```python
from build123d import *

# Parameters (mm, degrees)
F0_W     = 116
F0_H     = 156
F0_W_2   = 92
F0_H_2   = 132
F1_DEPTH = 12
F3_DEPTH = 116
F4_R     = 5
F5_R     = 15


with BuildPart() as f1:
    # F0 (on Top) → F1 (new body)
    with BuildSketch(Plane.XY):
        Rectangle(F0_W, F0_H)
        Rectangle(F0_W_2, F0_H_2, mode=Mode.SUBTRACT)
    extrude(amount=F1_DEPTH)

    # F2 (on face) → F3 (cut, through all)
    with BuildSketch(Plane(origin=(-58, 0, 0), x_dir=(0, -1, 0), z_dir=(-1, 0, 0))):
        Polygon((-78, 12), (78, 4), (78, 12), align=None)
    extrude(amount=-F3_DEPTH, mode=Mode.SUBTRACT)

    # F4
    f4_edges = [f1.edges().sort_by_distance(p)[0] for p in [
        (46, 66, 5.692308),
        (-46, 66, 5.692308),
        (-46, -66, 2.307692),
        (46, -66, 2.307692),
    ]]
    fillet(f4_edges, radius=F4_R)

    # F5
    f5_edges = [f1.edges().sort_by_distance(p)[0] for p in [
        (58, -78, 2),
        (-58, -78, 2),
        (-58, 78, 6),
        (58, 78, 6),
    ]]
    fillet(f5_edges, radius=F5_R)


solid = f1.part
```
Model file for the job. Use its own axes, mm. A direction names the side the tool comes from. Coordinates: 2 decimals unless noted, no trailing zeros. Order: outer loops, then holes, each group sorted by start corner. A loop starts at its lowest first (then second) coordinate and runs counter-clockwise, first axis right, second up. Notation, with made-up numbers: (69.5, 66.5) - (80.5, 66.5) arc R14 cw to (80.5, 82.5) - close; hole circle Ø4 at (13, 23). An arc over 180 degrees is marked (long way). Return JSON: item names as keys, results as strings. Group by question number.
1) Tool access for faces 4 (the cylindrical face through (-53.72, 73.49, 6.08)), 5 (the cylindrical face through (-44, -65, 2)): list every direction of +Z, -Z, +X, -X, +Y, -Y with a clear straight run to the whole face (end or side of a thin tool).
2) Probe line 1 (Y direction, x = 30, z = 2.25); line 2 (X direction, y = 56, z = 8.5); line 3 (Y direction, x = -31, z = 8.25). List the from-to ranges inside material, lowest first. Write a range as from..to.
3) Saw through at B-B, the plane y = -16. Write the cut outline in (x, z), plus the area to 3 significant figures.
4) Saw through at C-C, the plane x = 50. Write the cut outline in (y, z), plus the area to 3 significant figures.
5) Mould opens along Y. For faces 1 (the flat face through (58, 13, 4)), 2 (the cylindrical face through (53.49, -73.72, 2.42)), 3 (the cylindrical face through (45, 64, 6)) say: released by +Y, released by -Y, zero draft, split by the parting line, or undercut.
6) Saw through at A-A, the plane x = 21. Write the cut outline in (y, z), plus the area to 3 significant figures.
Values found:
{
 "1": {"face 4": "+Z, -Z, -X, +Y", "face 5": "+Z, -Z"},
 "2": {"line 1": "y = -78..-66, 66..78", "line 2": "x = -58..-46, 46..58", "line 3": "y = 66..78"},
 "3": {"outline": "(-58, 0) - (-46, 0) - (-46, 7.18) - (-58, 7.18) - close; (46, 0) - (58, 0) - (58, 7.18) - (46, 7.18) - close", "area": "172 mm²"},
 "4": {"outline": "(-76.27, 0) - (76.27, 0) - (76.27, 11.91) - (-76.27, 4.09) - close", "area": "1,220 mm²"},
 "5": {"face 1": "zero draft", "face 2": "released by -Y", "face 3": "undercut"},
 "6": {"outline": "(-78, 0) - (-66, 0) - (-66, 4.62) - (-78, 4) - close; (66, 0) - (78, 0) - (78, 12) - (66, 11.38) - close", "area": "192 mm²"}
}
